from build123d import *

# Parameters (mm, degrees)
F2_W = 3.175
F2_H = 3.175


with BuildPart() as f3:
    # F3: sweep along a path in F0
    with BuildLine(Plane.XY) as f3_path:
        Line((-147.2948789597, -61.8483945727), (-147.2948789597, -11.8481973186))
        Line((-147.2948789597, -11.8481973186), (-91.4910789597, -11.8481973186))
        Line((-91.4910789597, -11.8481973186), (-91.4910789597, -61.8483945727))
        Line((-91.4910789597, -61.8483945727), (-147.2948789597, -61.8483945727))
    # F2 (on line) → F3 (sweep)
    with BuildSketch(Plane(origin=(0, -61.8483945727, 0), x_dir=(-1, 0, 0), z_dir=(0, 1, 0))):
        with Locations((147.2948789597, 0)):
            Rectangle(F2_W, F2_H)
    sweep(path=f3_path.line, transition=Transition.RIGHT)


solid = f3.part
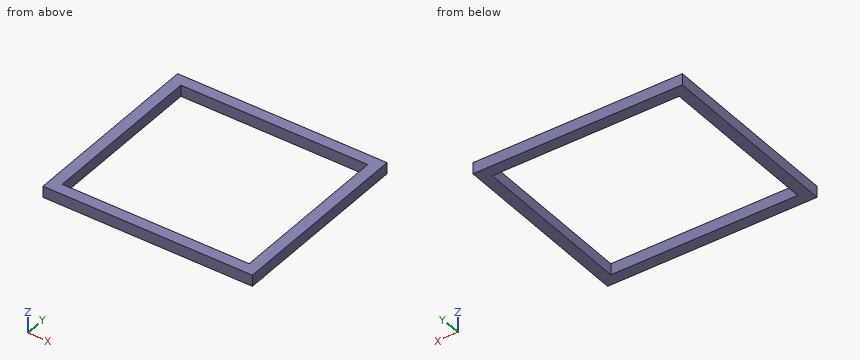
Check sheet for the modelled part. Datum: model origin and axes. Units: mm. Give positions to 0.01 mm unless a question says otherwise; leave off trailing zeros. Loops run counter-clockwise (first coordinate to the right, second up) from the corner with the lowest first, then second, coordinate; pieces in that order, holes last. Notation, with made-up numbers: M 84.25,53 L 132.25,53 A14 ccw 132.25,67 Z; hole C -37.5,65 d10. An arc over 180 degrees is marked long. Use a Markdown table: item, result. Add a question column.
Q1. Sectioned sample at B-B, the plane x = -136.5. Record the cut outline in (y, z), then the cut area to 3 significant figures.
Q2. Sectioned sample at C-C, the plane z = -0.45. Record the cut outline in (x, y), then the cut area to 3 significant figures.
Q3. Sectioned sample at A-A, the plane y = -21.5. Record the cut outline in (x, z).
Q4. Scan lines: line 1 along Y through (x, z) = (-122, -0.8); line 2 along X through (y, z) = (-40, -1.3). Record each from-to range of solid material in increasing order. Write a range as [from, to].
Verdict:
| question | item | result |
|---|---|---|
| 1 | outline | M -63.44,-1.59 L -60.26,-1.59 L -60.26,1.59 L -63.44,1.59 Z; M -13.44,-1.59 L -10.26,-1.59 L -10.26,1.59 L -13.44,1.59 Z |
| 1 | area | 20.2 mm^2 |
| 2 | outline | M -148.88,-63.44 L -89.9,-63.44 L -89.9,-10.26 L -148.88,-10.26 Z; hole M -145.71,-60.26 L -93.08,-60.26 L -93.08,-13.44 L -145.71,-13.44 Z |
| 2 | area | 672 mm^2 |
| 3 | outline | M -148.88,-1.59 L -145.71,-1.59 L -145.71,1.59 L -148.88,1.59 Z; M -93.08,-1.59 L -89.9,-1.59 L -89.9,1.59 L -93.08,1.59 Z |
| 4 | line 1 | [-63.44, -60.26], [-13.44, -10.26] |
| 4 | line 2 | [-148.88, -145.71], [-93.08, -89.9] |
